```python
from build123d import *

# Parameters (mm, degrees)
SKETCH_1_R               = 5
SKETCH_1_R_2             = 4
EXTRUDE_1_DEPTH          = 836.5
CUT_EXTRUDE_1_DEPTH      = 837.529885898
CUT_EXTRUDE_1_DEPTH_BACK = 837.529885898
SKETCH_2_R               = 2
SKETCH_2_R_2             = 1.5
SKETCH_2_3_R             = 4
SKETCH_2_3_R_2           = 3
CUT_EXTRUDE_2_DEPTH      = 837.529885999
CUT_EXTRUDE_3_DEPTH      = 837.529885999
CUT_EXTRUDE_3_DEPTH_BACK = 837.529885999
SKETCH_3_R               = 1.5
SKETCH_3_3_R             = 3
CUT_EXTRUDE_4_DEPTH      = 10


with BuildPart() as part:
    # Sketch 1 → Extrude 1 (new body)
    with BuildSketch(Plane.XY):
        Circle(SKETCH_1_R)
        Circle(SKETCH_1_R_2, mode=Mode.SUBTRACT)
    extrude(amount=EXTRUDE_1_DEPTH)

    # Sketch 2 → Cut-Extrude 1 (cut, two sides: drawn at the far end of the back side and taken through both)
    with BuildSketch(Plane(origin=(0, 0, 0), x_dir=(1, 0, 0), z_dir=(0, 1, 0)).offset(-CUT_EXTRUDE_1_DEPTH_BACK)):
        with Locations(Location((0, -820.5, 0), (0, 0, 270))):
            Circle(SKETCH_2_R)
        with Locations(Location((0, -797.5, 0), (0, 0, 270))):
            Circle(SKETCH_2_R_2)
    extrude(amount=CUT_EXTRUDE_1_DEPTH + CUT_EXTRUDE_1_DEPTH_BACK, mode=Mode.SUBTRACT)

    # Sketch 2_3 → Cut-Extrude 2 (cut, through all)
    with BuildSketch(Plane(origin=(0, 0, 0), x_dir=(1, 0, 0), z_dir=(0, 1, 0))):
        with Locations(Location((0, -820.5, 0), (0, 0, 90))):
            Circle(SKETCH_2_3_R)
        with Locations(Location((0, -797.5, 0), (0, 0, 90))):
            Circle(SKETCH_2_3_R_2)
    extrude(amount=CUT_EXTRUDE_2_DEPTH, mode=Mode.SUBTRACT)

    # Sketch 3 → Cut-Extrude 3 (cut, two sides: drawn at the far end of the back side and taken through both)
    with BuildSketch(Plane(origin=(0, 0, 0), x_dir=(0, 0, -1), z_dir=(1, 0, 0)).offset(-CUT_EXTRUDE_3_DEPTH_BACK)):
        with Locations((-48, 0)):
            Circle(SKETCH_3_R)
    extrude(amount=CUT_EXTRUDE_3_DEPTH + CUT_EXTRUDE_3_DEPTH_BACK, mode=Mode.SUBTRACT)

    # Sketch 3_3 → Cut-Extrude 4 (cut)
    with BuildSketch(Plane(origin=(0, 0, 0), x_dir=(0, 0, -1), z_dir=(1, 0, 0))):
        with Locations(Location((-48, 0, 0), (0, 0, 180))):
            Circle(SKETCH_3_3_R)
    extrude(amount=CUT_EXTRUDE_4_DEPTH, mode=Mode.SUBTRACT)


solid = part.part
```
Work out the finished part from the listing and answer in its coordinate system (mm). Give positions to 0.01 mm unless a question says otherwise; leave off trailing zeros. Write each loop counter-clockwise with the first axis right and the second up, starting at its lowest first coordinate (ties: lowest second). Pieces come first, ordered by that corner, then holes. Notation, with made-up numbers: (53.25, -31.75) -> (83.25, -31.75) arc R17 cw to (83.25, -1.75) -> close; hole circle Ø2 at (35.25, 72.5). An arc over 180 degrees is marked (long way). Write item = value, one per line.
Q1. Section B-B on z = 708 is taken. Determine the outline of the cut face in (x, y), and give its area (3 significant figures).
Computed values:
outline = circle Ø10 at (0, 0); hole circle Ø8 at (0, 0)
area = 28.3 mm^2
Q2. Flat-ended cylindrical pins translate along their axes: pin 1 Ø1.5 at (y, z) = (-2, 334.5) entering from +X; pin 2 Ø3 at (y, z) = (1.5, 303.5) entering from -X; pin 3 Ø1.5 at (y, z) = (-2, 626.5) entering from -X; pin 4 Ø5 at (y, z) = (0, 48) entering from +X. Find the tip coordinate at first contact, or state that the pin passes through.
Computed values:
pin_1 = 4.84
pin_2 = -5
pin_3 = -4.84
pin_4 = -3.12
Q3. Consider line 1 along Z through (x, y) = (0, -4.45); line 2 along Y through (x, z) = (-0.25, 374); line 3 along Y through (x, z) = (-0.75, 357.5). Determine where each line is inside the solid, lowest interval first.
Computed values:
line_1 = 0 to 796, 799 to 818.5, 822.5 to 836.5
line_2 = -4.99 to -3.99, 3.99 to 4.99
line_3 = -4.94 to -3.93, 3.93 to 4.94
Q4. Section A-A on x = 0 is taken. Determine the outline of the cut face in (y, z), and give its area (3 significant figures).
Computed values:
outline = (-5, 0) -> (-4, 0) -> (-4, 796) -> (-5, 796) -> close; (-5, 799) -> (-4, 799) -> (-4, 818.5) -> (-5, 818.5) -> close; (-5, 822.5) -> (-4, 822.5) -> (-4, 836.5) -> (-5, 836.5) -> close; (4, 0) -> (5, 0) -> (5, 794.5) -> (4, 794.5) -> close; (4, 800.5) -> (5, 800.5) -> (5, 816.5) -> (4, 816.5) -> close; (4, 824.5) -> (5, 824.5) -> (5, 836.5) -> (4, 836.5) -> close
area = 1,650 mm^2
